```python
from build123d import *

# Parameters (mm, degrees)
F1_DEPTH = 1


# Not quite as in the source:
# - a feature names something its author has since deleted; it is built from what else it names


with BuildPart() as f1:
    # F0 (on Top) → F1 (new body)
    with BuildSketch(Plane.XY):
        with BuildLine():
            Line((-2.7494849637, -25.4823859731), (-2.7494849637, -25.250749146))
            ThreePointArc((-2.7494849637, -25.250749146), (-22.497868801, -11.7900763108), (-22.3279049811, 12.1088669642))
            Line((-22.3279049811, 12.1088669642), (-38.057784897, -16.8959317215))
            ThreePointArc((-38.057784897, -16.8959317215), (-37.8884434924, -23.2436733268), (-32.3064673032, -26.2708901713))
            Line((-32.3064673032, -26.2708901713), (-2.7494849637, -25.4823859731))
        make_face()
        with BuildLine():
            ThreePointArc((25.4, 0), (19.4537790742, -16.3312730591), (4.3991748244, -25.0161400073))
            Line((4.3991748244, -25.0161400073), (4.3991748244, -25.2916781332))
            Line((4.3991748244, -25.2916781332), (33.6611985399, -24.5110426718))
            ThreePointArc((33.6611985399, -24.5110426718), (39.0738333245, -21.1905179108), (38.9044919199, -14.8427763054))
            Line((38.9044919199, -14.8427763054), (21.6505391613, 13.2820990068))
            ThreePointArc((21.6505391613, 13.2820990068), (24.4446690988, 6.9005907466), (25.4, 0))
        make_face()
        with BuildLine():
            ThreePointArc((-22.3279049811, 12.1088669642), (-22.497868801, -11.7900763108), (-2.7494849637, -25.250749146))
            ThreePointArc((-2.7494849637, -25.250749146), (0.8331443579, -25.3863323558), (4.3991748244, -25.0161400073))
            ThreePointArc((4.3991748244, -25.0161400073), (19.4537790742, -16.3312730591), (25.4, 0))
            ThreePointArc((25.4, 0), (24.4446690988, 6.9005907466), (21.6505391613, 13.2820990068))
            ThreePointArc((21.6505391613, 13.2820990068), (-0.6773658317, 25.3909664158), (-22.3279049811, 12.1088669642))
        make_face()
        with BuildLine():
            Line((-3.4520485887, 46.9146262965), (-22.3279049811, 12.1088669642))
            ThreePointArc((-22.3279049811, 12.1088669642), (-0.6773658317, 25.3909664158), (21.6505391613, 13.2820990068))
            Line((21.6505391613, 13.2820990068), (0.9457958008, 47.0319494631))
            ThreePointArc((0.9457958008, 47.0319494631), (-1.2869946749, 48.2428362009), (-3.4520485887, 46.9146262965))
        make_face()
        with BuildLine():
            ThreePointArc((4.3991748244, -25.0161400073), (0.8331443579, -25.3863323558), (-2.7494849637, -25.250749146))
            Line((-2.7494849637, -25.250749146), (-2.7494849637, -25.4823859731))
            Line((-2.7494849637, -25.4823859731), (-2.7494849637, -40.7840199769))
            Line((-2.7494849637, -40.7840199769), (4.3991748244, -40.7840199769))
            Line((4.3991748244, -40.7840199769), (4.3991748244, -25.2916781332))
            Line((4.3991748244, -25.2916781332), (4.3991748244, -25.0161400073))
        make_face()
    extrude(amount=F1_DEPTH)


solid = f1.part
```
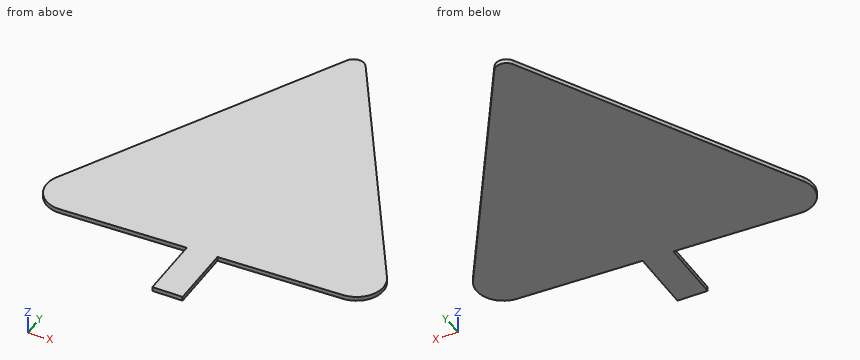
For this review, take the finished solid that the model builds, in its own axes (mm). Coordinates: 2 decimals unless noted, no trailing zeros. Loops run counter-clockwise (first coordinate to the right, second up) from the corner with the lowest first, then second, coordinate; pieces in that order, holes last.
1. Add section B-B, the plane y = -27.5. Give the boundary of the cut face in (x, z).
2. Add section A-A, the plane z = 0.3. Give the boundary of the cut face in (x, y), then the cut area to 3 significant figures.
3. For line 1 (X direction, y = -36, z = 0.9); line 2 (X direction, y = 0.5, z = 0.35); line 3 (Y direction, x = 10, z = 0.5), list the stretches that pass through material, from the lowest coordinate up.
4. Add section C-C, the plane x = -29. Give the boundary of the cut face in (y, z), then the cut area to 3 significant figures.
Result:
1. outline: (-2.75, 0) - (4.4, 0) - (4.4, 1) - (-2.75, 1) - close
2. outline: (-38.06, -16.9) arc R6.35 ccw to (-32.31, -26.27) - (-2.75, -25.48) - (-2.75, -40.78) - (4.4, -40.78) - (4.4, -25.29) - (33.66, -24.51) arc R6.35 ccw to (38.9, -14.84) - (0.95, 47.03) arc R2.54 ccw to (-3.45, 46.91) - close
2. area: 3,400 mm2
3. line 1: x = -2.75 to 4.4
3. line 2: x = -28.62 to 29.49
3. line 3: y = -25.14 to 32.27
4. outline: (-26.18, 0) - (-0.19, 0) - (-0.19, 1) - (-26.18, 1) - close
4. area: 26.0 mm2
